from build123d import *

# Parameters (mm, degrees)
F1_DEPTH = 114.3
F2_R     = 50.8
F3_R     = 25.4


with BuildPart() as f1:
    # F0 (on Top) → F1 (new body)
    with BuildSketch(Plane.XY):
        with BuildLine():
            Line((-42.803083, -177.8), (-305.849485, -177.8))
            ThreePointArc((-305.849485, -177.8), (-50.599354, -317.404266), (211.196917, -190.5))
            Line((211.196917, -190.5), (1016, -190.5))
            ThreePointArc((1016, -190.5), (1270, -317.5), (1524, -190.5))
            Line((1524, -190.5), (1270, -190.5))
            ThreePointArc((1270, -190.5), (1096.116526, 0), (1270, 190.5))
            Line((1270, 190.5), (1524, 190.5))
            ThreePointArc((1524, 190.5), (1270, 317.5), (1016, 190.5))
            Line((1016, 190.5), (211.196917, 190.5))
            ThreePointArc((211.196917, 190.5), (-50.599354, 317.404266), (-305.849485, 177.8))
            Line((-305.849485, 177.8), (-42.803083, 177.8))
            ThreePointArc((-42.803083, 177.8), (-34.172165, 178.009361), (-25.541248, 177.8))
            ThreePointArc((-25.541248, 177.8), (143.837196, 0), (-25.541248, -177.8))
            ThreePointArc((-25.541248, -177.8), (-34.172165, -178.009361), (-42.803083, -177.8))
        make_face()
        with BuildLine():
            Line((-25.541248, -177.8), (-42.803083, -177.8))
            ThreePointArc((-42.803083, -177.8), (-34.172165, -178.009361), (-25.541248, -177.8))
        make_face()
        with BuildLine():
            Line((-42.803083, 177.8), (-25.541248, 177.8))
            ThreePointArc((-25.541248, 177.8), (-34.172165, 178.009361), (-42.803083, 177.8))
        make_face()
    extrude(amount=F1_DEPTH)

    # F2
    f2_edges = [f1.edges().sort_by_distance(p)[0] for p in [
        (211.196917, 190.5, 57.15),
        (1016, 190.5, 57.15),
        (211.196917, -190.5, 57.15),
        (1016, -190.5, 57.15),
    ]]
    fillet(f2_edges, radius=F2_R)

    # F3
    f3_edges = [f1.edges().sort_by_distance(p)[0] for p in [
        (-305.849485, 177.8, 57.15),
        (-305.849485, -177.8, 57.15),
        (1524, 190.5, 57.15),
        (1524, -190.5, 57.15),
    ]]
    fillet(f3_edges, radius=F3_R)


solid = f1.part
Can you work these out from the model? Positions are in its coordinate system, mm. A direction names the side the tool comes from. Coordinates: 2 decimals unless noted, no trailing zeros. Loops run counter-clockwise (first coordinate to the right, second up) from the corner with the lowest first, then second, coordinate; pieces in that order, holes last. Notation, with made-up numbers: (32.5, -21) - (70.5, -21) arc R12 ccw to (70.5, -1) - close; hole circle Ø2 at (38.5, 38). An arc over 180 degrees is marked (long way). Put each result on its own line as item: value. Start each with the question number.
Item 1: Suppose I cut it at D-D (y = 0). Please give me the cut outline in (x, z), and give its area (3 significant figures).
Item 2: Suppose I cut it at C-C (y = -262). Please give me the cut outline in (x, z), and give its area (3 significant figures).
Item 3: Which directions (+Z, -Z, +X, -X, +Y, -Y) give clear straight access to the entire face, cutting with the end or side of a thin tool? Please do faces 1 (the face through (1367, 190.5, 56)), 2 (the face through (1012.57, -194.96, 57.95)), 3 (the face through (-138, -177.8, 56)).
Item 4: Suppose I cut it at A-A (z = 48). Please give me the cut outline in (x, y).
Item 5: If I drill on line 1 along Y through (x, z) = (740.5, 94.5); line 2 along X through (y, z) = (203, 84); line 3 along Y through (x, z) = (1388, 10), over which ranges is the centre line in solid material (lowest first)?
Item 6: Suppose I cut it at B-B (x = 1301.5). Please give me the cut outline in (y, z), and give its area (3 significant figures).
Item 7: If we mould it in two halves opening along Y, with no side actions, what happens to faces 4 (the face through (1254.92, 317.14, 56.35)), 5 (the face through (214.1, -195.2, 58)), 6 (the face through (-141, 177.8, 56))? For each: +Y half, -Y half, draft (parallel to the pull), parting line (faces both ways), or undercut.
Item 8: For pin 1 (10 mm diameter, centred on y = 191, z = 63, fed in from +X); pin 2 (6 mm diameter, centred on y = 182, z = 38, fed in from -X); pin 3 (1 mm diameter, centred on x = 1258, y = -187, fed in from -Z); pin 4 (5 mm diameter, centred on y = 199.5, z = 56.5, fed in from -X), each with a flat end and sliding along its axis, tell me the tip position at first contact or that it passes through.
Here are the results:
1. outline: (143.84, 0) - (1096.12, 0) - (1096.12, 114.3) - (143.84, 114.3) - close
1. area: 109,000 mm²
2. outline: (-222.14, 0) - (136.54, 0) - (136.54, 114.3) - (-222.14, 114.3) - close; (1090.66, 0) - (1449.34, 0) - (1449.34, 114.3) - (1090.66, 114.3) - close
2. area: 82,000 mm²
3. face 1: +Z, -Z, +X
3. face 2: +Z, -Z, -Y
3. face 3: +Z, -Z, -X
4. outline: (-270.89, -220.87) arc R317.5 ccw to (197.06, -208.02) arc R50.8 cw to (235.44, -190.5) - (991.76, -190.5) arc R50.8 cw to (1030.14, -208.02) arc R317.5 ccw to (1483.86, -234.67) arc R25.4 ccw to (1466.75, -190.5) - (1270, -190.5) arc R191.29 cw to (1270, 190.5) - (1466.75, 190.5) arc R25.4 ccw to (1483.86, 234.67) arc R317.5 ccw to (1030.14, 208.02) arc R50.8 cw to (991.76, 190.5) - (235.44, 190.5) arc R50.8 cw to (197.06, 208.02) arc R317.5 ccw to (-270.89, 220.87) arc R25.4 ccw to (-252.64, 177.8) - (-25.54, 177.8) arc R178.01 cw to (-25.54, -177.8) - (-252.64, -177.8) arc R25.4 ccw to start
5. line 1: -190.5 to 190.5
5. line 2: -278.04 to 202.07, 1025.13 to 1488.63
5. line 3: -294.76 to -190.5, 190.5 to 294.76
6. outline: (-315.93, 0) - (-190.5, 0) - (-190.5, 114.3) - (-315.93, 114.3) - close; (190.5, 0) - (315.93, 0) - (315.93, 114.3) - (190.5, 114.3) - close
6. area: 28,700 mm²
7. face 4: +Y half
7. face 5: -Y half
7. face 6: undercut
8. pin 1: x = 1482.53
8. pin 2: x = -270.36
8. pin 3: through
8. pin 4: x = -278.01
